Part model, mm, in its own coordinate system. Face numbers are marked on the shaded views. A direction names the side the tool comes from. Coordinates: 2 decimals unless noted, no trailing zeros. Order: outer loops, then holes, each group sorted by start corner. A loop starts at its lowest first (then second) coordinate and runs counter-clockwise, first axis right, second up.
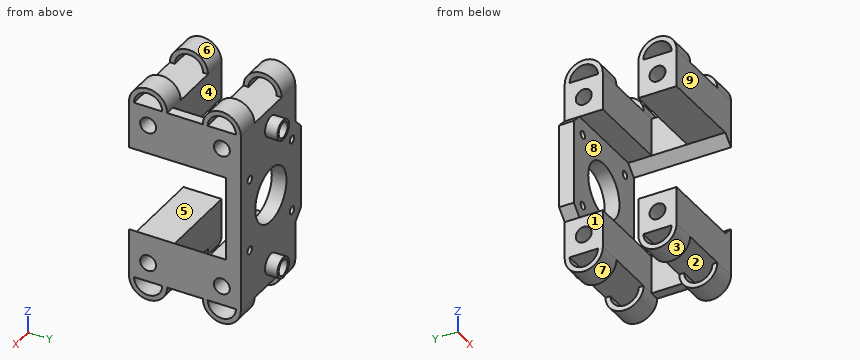
Autodesk Inventor part; units mm, degrees
ref_plane "Work Plane1" through (0, -16.75, 0) normal (0, -1, 0) x (1, 0, 0)
ref_plane "Work Plane2" through (-17.25, 6, 0) normal (0, 0, 1) x (1, 0, 0)
ref_plane "Work Plane3" through (2, 6, 36.75) normal (1, 0, 0) x (0, 0, -1)
sketch "Sketch1" plane through (0, 0, 0) normal (0, 1, 0) x (-1, 0, 0)
  circle A0 centre (0, 0) radius 11.05
  line L0 (17.25, 21.25) -> (21.25, 17.25)
  line L1 (21.25, 17.25) -> (21.25, -17.25)
  line L2 (21.25, -17.25) -> (17.25, -21.25)
  line L3 (17.25, -21.25) -> (-17.25, -21.25)
  line L4 (-17.25, -21.25) -> (-21.25, -17.25)
  line L5 (-21.25, -17.25) -> (-21.25, 17.25)
  line L6 (-21.25, 17.25) -> (-17.25, 21.25)
  line L7 (-17.25, 21.25) -> (17.25, 21.25)
  line L8 (0, 21.25) -> (0, -21.25) construction
  line L9 (21.25, 0) -> (-21.25, 0) construction
  circle A1 centre (14.8987, 14.8987) radius 1.55
  line L10 (14.8987, 14.8987) -> (0, 0) construction
  circle A2 centre (-14.8987, 14.8987) radius 1.55
  circle A3 centre (-14.8987, -14.8987) radius 1.55
  circle A4 centre (14.8987, -14.8987) radius 1.55
  dimension "d0" = 22.1
  dimension "d1" = 42.5
  dimension "d2" = 4
  dimension "d3" = 135
  dimension "d4" = 3.1
  dimension "d5" = 21.07
  dimension "d6" = 45
  dimension "d9" = 360
extrude "Extrusion1" add sketch "Sketch1" along normal blind 6
sketch "Sketch2" plane through (0, 6, 0) normal (0, 1, 0) x (1, 0, 0)
  line L0 (-21.25, -17.25) -> (-17.25, -21.25)
  line L1 (-17.25, -21.25) -> (-17.25, -36.75)
  line L2 (-17.25, -36.75) -> (21.25, -36.75)
  line L3 (21.25, -36.75) -> (21.25, 36.75)
  line L4 (21.25, 36.75) -> (-17.25, 36.75)
  line L5 (17.25, 21.25) -> (-17.25, 21.25)
  line L6 (-17.25, 36.75) -> (-17.25, 21.25)
  line L7 (-17.25, 21.25) -> (17.25, 21.25)
  line L8 (21.25, 17.25) -> (17.25, 21.25)
  line L9 (17.25, 21.25) -> (21.25, 17.25)
  line L10 (21.25, 17.25) -> (21.25, -17.25)
  line L11 (21.25, -17.25) -> (17.25, -21.25)
  line L12 (17.25, -21.25) -> (-17.25, -21.25)
  line L13 (21.25, -17.25) -> (21.25, 17.25)
  point P0 (0, 0)
  point P1 (21.25, -17.25)
  dimension "d13" = 15.5
extrude "Extrusion2" add sketch "Sketch2" against normal blind 15.5
sketch "Sketch3" plane through (0, -9.5, 0) normal (0, -1, 0) x (1, 0, 0)
  line L0 (21.25, 36.75) -> (21.25, -36.75)
  line L1 (21.25, -17.25) -> (17.25, -21.25)
  line L2 (21.25, -36.75) -> (21.25, -17.25)
  line L3 (21.25, -17.25) -> (17.25, -21.25)
  line L4 (17.25, -21.25) -> (17.25, -36.75)
  line L5 (17.25, -36.75) -> (21.25, -36.75)
  line L6 (17.25, 21.25) -> (21.25, 17.25)
  line L7 (21.25, 17.25) -> (17.25, 21.25)
  line L8 (17.25, 21.25) -> (17.25, 36.75)
  line L9 (21.25, 36.75) -> (-17.25, 36.75)
  line L10 (21.25, 36.75) -> (21.25, 17.25)
  point P0 (0, 0)
extrude "Extrusion3" add sketch "Sketch3" along normal blind 30
sketch "Sketch4" plane through (17.25, -9.5, 21.25) normal (-1, 0, 0) x (0, 0, 1)
  line L0 (15.5, 15.5) -> (15.5, -30)
  line L1 (0, 0) -> (0, -30)
  line L2 (15.5, -30) -> (0, -30)
  line L3 (0, -30) -> (0, -14.5)
  line L4 (0, -14.5) -> (15.5, -14.5)
  line L5 (15.5, -14.5) -> (15.5, -30)
  line L6 (-42.5, 0) -> (-42.5, -30)
  line L7 (-58, 15.5) -> (-58, -30)
  line L8 (-42.5, -30) -> (-58, -30)
  line L9 (-58, -30) -> (-58, -14.5)
  line L10 (-58, -14.5) -> (-42.5, -14.5)
  line L11 (-42.5, -14.5) -> (-42.5, -30)
  point P0 (-21.25, 9.5)
  point P1 (0, -30)
  point P2 (15.5, -14.5)
  dimension "d18" = 15.5
extrude "Extrusion4" add sketch "Sketch4" along normal up to surface (34.5 mm away)
sketch "Sketch5" plane through (-17.25, -39.5, -21.25) normal (-1, 0, 0) x (0, 0, 1)
  line L0 (-15.5, 15.5) -> (0, 15.5) construction
  line L1 (-7.75, 15.5) -> (-7.75, 0) construction
  line L2 (-15.5, 0) -> (4, 0) construction
  circle A0 centre (-7.75, 7.75) radius 3.25
  line L3 (-15.5, 0) -> (-15.5, 15.5) construction
  line L4 (-15.5, 7.75) -> (-7.75, 7.75) construction
  circle A1 centre (-7.75, 37.75) radius 3.25
  circle A2 centre (50.25, 7.75) radius 3.25
  circle A3 centre (50.25, 37.75) radius 3.25
  point P0 (21.25, 39.5)
  dimension "d21" = 6.5
  dimension "d24" = 30
  dimension "d27" = 58
extrude "Extrusion5" cut sketch "Sketch5" against normal up to surface (38.5 mm away)
sketch "Sketch6" plane through (-17.25, -39.5, 36.75) normal (-1, 0, 0) x (0, 0, 1)
  arc A0 (0, 2) -> (0, 13.5) centre (0, 7.75) ccw
  arc A1 (0, 0) -> (0, 15.5) centre (0, 7.75) ccw
  line L0 (0, 0) -> (0, 2)
  line L1 (0, 13.5) -> (0, 15.5)
  line L2 (0, 15.5) -> (0, 0)
  point P0 (-36.75, 39.5)
  dimension "d32" = 2
  dimension "d34" = 180
extrude "Extrusion6" add sketch "Sketch6" against normal up to surface (38.5 mm away) contours A0 L1 A1 L0
ref_plane "Work Plane1" through (0, -16.75, 0) normal (0, -1, 0) x (1, 0, 0)
ref_plane "Work Plane2" through (-17.25, 6, 0) normal (0, 0, 1) x (1, 0, 0)
ref_plane "Work Plane3" through (2, 6, 36.75) normal (1, 0, 0) x (0, 0, -1)
mirror "Mirror1" about plane through (0, -16.75, 0) normal (0, -1, 0) of "Extrusion6"
mirror "Mirror2" about plane through (-17.25, 6, 0) normal (0, 0, 1) of "Extrusion6", "Mirror1"
sketch "Sketch7" plane through (2, 6, 36.75) normal (1, 0, 0) x (0, 0, -1)
  line L0 (19.5, -45.5) -> (0, -45.5)
  line L1 (0, -45.5) -> (-7.75, -45.5)
  line L2 (-7.75, -45.5) -> (-7.75, 0)
  line L3 (-7.75, 0) -> (0, 0)
  line L4 (0, 0) -> (0, -45.5)
  arc A0 (0, -30) -> (0, -45.5) centre (0, -37.75) ccw
  arc A1 (73.5, -45.5) -> (73.5, -30) centre (73.5, -37.75) ccw
  line L5 (73.5, -45.5) -> (81.25, -45.5)
  line L6 (81.25, -45.5) -> (81.25, 0)
  line L7 (81.25, 0) -> (73.5, 0)
  line L8 (73.5, 0) -> (73.5, -45.5)
  point P0 (36.75, -6)
  point P1 (19.5, 0)
extrude "Extrusion7" cut sketch "Sketch7" along normal mid plane 19.25
sketch "Sketch8" plane through (0, 6, 0) normal (0, 1, 0) x (1, 0, 0)
  line L0 (17.25, -36.75) -> (-17.25, -36.75) construction
  line L1 (21.25, 36.75) -> (-17.25, 36.75) construction
  line L2 (-17.25, -21.25) -> (-17.25, -36.75) construction
  line L3 (-17.25, -21.25) -> (17.25, -21.25) construction
  line L4 (-17.25, -36.75) -> (21.25, -36.75) construction
  line L5 (21.25, -36.75) -> (21.25, -21.25) construction
  line L6 (21.25, -21.25) -> (-17.25, -21.25) construction
  line L7 (-17.25, -21.25) -> (-17.25, -36.75) construction
  line L8 (21.25, -36.75) -> (21.25, 36.75) construction
  line L9 (0, -36.75) -> (0, -21.25) construction
  circle A0 centre (0, -29) radius 3.15
  circle A1 centre (0, -29) radius 4.15
  point P0 (0, 0)
  point P1 (11.625, -36.75)
  point P2 (-7.625, -36.75)
  point P3 (11.625, 36.75)
  point P4 (-7.625, 36.75)
  dimension "d39" = 6.3
  dimension "d40" = 1
extrude "Extrusion8" add sketch "Sketch8" along normal blind 5
mirror "Mirror3" about plane through (-17.25, 6, 0) normal (0, 0, 1) of "Extrusion8"
equation "\"d11\" = mount_face_thickness"
equation "\"d13\" = post_width"
equation "\"d14\" = post_width"
equation "\"d16\" = mount_length - post_width"
equation "\"d18\" = post_width"
equation "\"d19\" = mount_length - post_width"
equation "\"d21\" = rod_diameter + rod_free_tolerance"
equation "\"d24\" = mount_length - post_width"
equation "\"d39\" = slider_rod_diameter + slider_rod_tolerance"
equation "\"mount_face_thickness\" = 6"
equation "\"post_width\" = 15.5"
equation "\"slider_rod_diameter\" = 6"
equation "\"rod_diameter\" = 6"
equation "\"rod_free_tolerance\" = 0.5"
equation "\"mount_length\" = 45.5"
equation "\"slider_rod_tolerance\" = 0.3"
properties part number "carriage_motor_mount"
Q1. Wall check: line 1 along Z through (x, y) = (-3, -1); line 2 along Y through (x, z) = (3, -29); line 3 along Z through (x, y) = (0, 9). Give the ranges that are in metal, low to high.
Results list:
line 1: z = -36.75 to -32.16, -25.84 to -21.25, 21.25 to 25.84, 32.16 to 36.75
line 2: y = -39.5 to -35, -28.5 to -24, -9.5 to -5, 1.5 to 6
line 3: z = -33.15 to -32.15, -25.85 to -24.85, 24.85 to 25.85, 32.15 to 33.15
Q2. Cut at B-B on z = 0. Write the cut outline in (x, y), and give its area (3 significant figures).
Results list:
outline: (-21.25, 0) - (-11.05, 0) - (-11.05, 6) - (-21.25, 6) - close; (11.05, 0) - (21.25, 0) - (21.25, 6) - (11.05, 6) - close
area: 122 mm2
Q3. Pin check, flat tips, straight feed: pin 1 Ø8.5 at (y, z) = (-31.5, -42) entering from -X; pin 2 Ø2.5 at (y, z) = (-35.5, -39) entering from +X; pin 3 Ø1.5 at (x, y) = (2.5, -26.5) entering from -Z; pin 4 Ø2 at (x, y) = (-6.5, -25) entering from +Z. Stop position of each tip, or through.
Results list:
pin 1: stops at x = -17.25
pin 2: passes through
pin 3: stops at z = -36.75
pin 4: stops at z = 36.75
Q4. Cut at A-A on y = -23. Write the cut outline in (x, z), and give its area (3 significant figures).
Results list:
outline: (17.25, -36.75) - (21.25, -36.75) - (21.25, -17.25) - (17.25, -21.25) - close; (17.25, 21.25) - (21.25, 17.25) - (21.25, 36.75) - (17.25, 36.75) - close
area: 140 mm2
Q5. Cut at D-D on y = -31.75. Count the separate pieces of the cut face and the enclosed holes in it, and give its area (3 significant figures).
Results list:
separate pieces: 8
enclosed holes: 0
area: 786 mm2
Q6. Mould opens along Z. For the marked faces 6, 7, 8 and 9 say: pulls with the +Z half, pulls with the -Z half, needs draft (parallel to the pull), parting line crosses it, or undercut.
Results list:
face 6: pulls with the +Z half
face 7: pulls with the -Z half
face 8: undercut
face 9: needs draft
Q7. Which spindle directions (+Z, -Z, +X, -X, +Y, -Y) get a long thin tool onto all of the face, cutting with end or side? Do the marked faces 1, 2, 3, 4 and 5. Say none if no direction does.
Results list:
face 1: -Z, -X, +Y, -Y
face 2: none
face 3: -Z, +X, -X
face 4: +Z, -Z, -X
face 5: -X, -Y
Q8. Cut at C-C on z = 29. Write the cut outline in (x, y).
Results list:
outline: (-17.25, -39.5) - (21.25, -39.5) - (21.25, -35) - (-17.25, -35) - close; (-17.25, -28.5) - (21.25, -28.5) - (21.25, -5) - (-17.25, -5) - (-17.25, -9.5) - (17.25, -9.5) - (17.25, -24) - (-17.25, -24) - close; (-17.25, 1.5) - (21.25, 1.5) - (21.25, 6) - (4.15, 6) - (4.15, 11) - (3.15, 11) - (3.15, 6) - (-3.15, 6) - (-3.15, 11) - (-4.15, 11) - (-4.15, 6) - (-17.25, 6) - close
